Check sheet for the drawn part. Datum: minimum x, y, z corner. Units: mm. A direction names the side the tool comes from. Give positions to 0.01 mm unless a question says otherwise; leave off trailing zeros. Order: outer loops, then holes, each group sorted by start corner. A loop starts at its lowest first (then second) coordinate and runs counter-clockwise, first axis right, second up. Notation, with made-up numbers: (11, 76) -> (60, 76) arc R32 ccw to (60, 109) -> close; hole circle Ø8 at (27, 71). An arc over 180 degrees is marked (long way). Return JSON: item names as keys, results as strings. Group by question number.
(1) Tool access check on the marked faces 4 and 5. Record the directions out of +Z, -Z, +X, -X, +Y, -Y that give a thin tool (end or side, any length) a straight path to the whole face; none if there is none.
(2) Cross-section at A-A on y = 52.8. Enter the section's corners in (x, z).
(3) Depth check by flat-ended pin: pin 1 Ø4 at (y, z) = (54, 4.5) entering from -X. Enter the tip coordinate at first touch or a pass-through.
(4) Cross-section at B-B on x = 13.2. Enter the section's corners in (y, z).
(5) Cross-section at C-C on z = 3.5. State how many separate pieces and enclosed holes the cut face has.
(6) Cross-section at D-D on x = 35.5. Enter the section's corners in (y, z) (1 decimal).
(7) Release check for a two-part mould opening along Y. For the marked faces 1, 2 and 3 record: pulls with the +Y half, pulls with the -Y half, needs draft (parallel to the pull), parting line crosses it, or undercut.
(8) Thickness scan on line 1 along Y through (x, z) = (36.5, 5.5); line 2 along X through (y, z) = (11, 5) (1 decimal); line 3 along Y through (x, z) = (13.2, 3.75). Record the ranges inside material, lowest first.
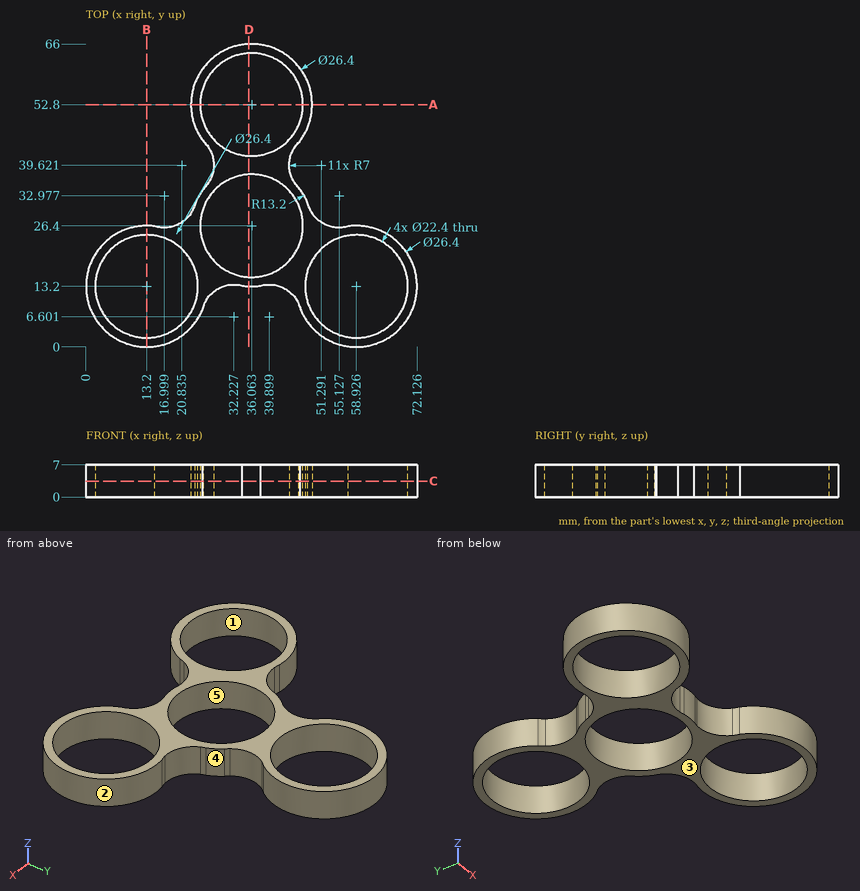
Verdict:
{
 "1": {"face 4": "+Z, -Z, +X", "face 5": "+Z, -Z"},
 "2": {"outline": "(22.86, 0) -> (24.86, 0) -> (24.86, 7) -> (22.86, 7) -> close; (47.26, 0) -> (49.26, 0) -> (49.26, 7) -> (47.26, 7) -> close"},
 "3": {"pin 1": "x = 22.86"},
 "4": {"outline": "(0, 0) -> (2, 0) -> (2, 7) -> (0, 7) -> close; (24.4, 0) -> (26.4, 0) -> (26.4, 7) -> (24.4, 7) -> close"},
 "5": {"separate pieces": "1", "enclosed holes": "4"},
 "6": {"outline": "(13.2, 0) -> (15.2, 0) -> (15.2, 7) -> (13.2, 7) -> close; (37.6, 0) -> (41.6, 0) -> (41.6, 7) -> (37.6, 7) -> close; (64, 0) -> (66, 0) -> (66, 7) -> (64, 7) -> close"},
 "7": {"face 1": "undercut", "face 2": "parting line crosses it", "face 3": "needs draft"},
 "8": {"line 1": "13.21 to 15.21, 37.59 to 41.61, 63.99 to 65.99", "line 2": "0.2 to 2.2, 24.2 to 26.8, 45.3 to 47.9, 69.9 to 71.9", "line 3": "0 to 2, 24.4 to 26.4"}
}
